The listing builds one solid part. Answer for the finished solid, in the listing's coordinates (mm). Coordinates: 2 decimals unless noted, no trailing zeros. Loops run counter-clockwise (first coordinate to the right, second up) from the corner with the lowest first, then second, coordinate; pieces in that order, holes last. Notation, with made-up numbers: (64.5, 51) - (96.5, 51) arc R17 ccw to (96.5, 78) - close; hole circle Ø3 at (66, 83). An arc over 180 degrees is marked (long way). Put each result on its own line as item: value.
```python
from build123d import *

# Parameters (mm, degrees)
F0_W          = 20
F0_H          = 75
F0_R          = 3.5
F1_DEPTH      = 1
F2_R          = 3
F3_DEPTH      = 75
F4_W          = 8
F4_H          = 15
F5_DEPTH      = 1.001
F5_DEPTH_BACK = 7.001


with BuildPart() as f1:
    # F0 (on Front) → F1 (new body)
    with BuildSketch(Plane.XZ):
        with Locations((-10, 0)):
            Rectangle(F0_W, F0_H)
        with Locations((-10, -26)):
            Circle(F0_R, mode=Mode.SUBTRACT)
        with Locations((-10, 0)):
            Circle(F0_R, mode=Mode.SUBTRACT)
        with Locations((-10, 26)):
            Circle(F0_R, mode=Mode.SUBTRACT)
    extrude(amount=F1_DEPTH)

    # F2 (on face) → F3 (join, through all)
    with BuildSketch(Plane(origin=(0, 0, -37.5), x_dir=(1, 0, 0), z_dir=(0, 0, -1))):
        with BuildLine():
            ThreePointArc((-20.8542486889, 1), (-19.8542486889, 2.3542486889), (-19.5, 4))
            ThreePointArc((-19.5, 4), (-26.3284271247, 6.8284271247), (-23.5, 0))
            ThreePointArc((-23.5, 0), (-22.0857864376, 0.2583426132), (-20.8542486889, 1))
        make_face()
        with Locations((-23.5, 4)):
            Circle(F2_R, mode=Mode.SUBTRACT)
        with BuildLine():
            ThreePointArc((-20.8542486889, 1), (-22.0857864376, 0.2583426132), (-23.5, 0))
            Line((-23.5, 0), (-20, 0))
            Line((-20, 0), (-20, 1))
            Line((-20, 1), (-20.8542486889, 1))
        make_face()
    extrude(amount=-F3_DEPTH)

    # F4 (on face) → F5 (cut, two sides)
    with BuildSketch(Plane.XZ.offset(1)) as f5_sk:
        with Locations((-23.5, 30)):
            Rectangle(F4_W, F4_H)
        with Locations((-23.5, -30)):
            Rectangle(F4_W, F4_H)
        with Locations((-23.5, 0)):
            Rectangle(F4_W, F4_H)
    extrude(amount=-F5_DEPTH, mode=Mode.SUBTRACT)
    extrude(f5_sk.sketch, amount=F5_DEPTH_BACK, mode=Mode.SUBTRACT)


solid = f1.part
```
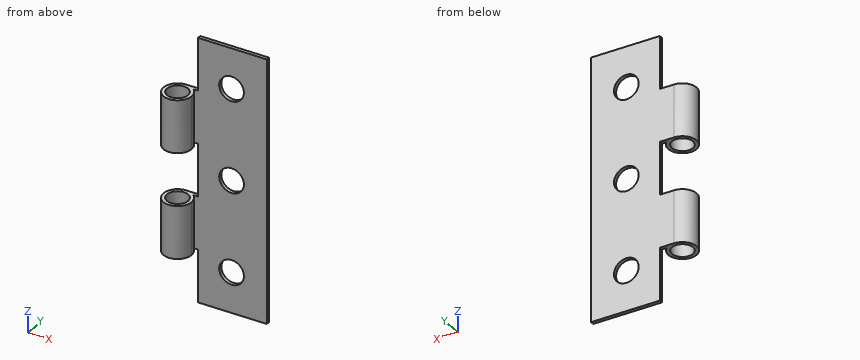
1) The part is cut by section D-D (z = 14). Give the vertices of the cut face in (x, y), and give its area (3 significant figures).
Found:
outline: (-23.5, 0) arc R4 ccw (long way) to (-20.85, -1) - (0, -1) - (0, 0) - close; hole circle Ø6 at (-23.5, -4)
area: 43.7 mm^2
2) Each of these flat-tipped pins is pushed along its axis until it touches: pin 1 (0.8 mm diameter, centred on y = -0.5, z = -31.5, fed in from -X); pin 2 (4 mm diameter, centred on x = -25, y = -4.5, fed in from -Z); pin 3 (4 mm diameter, centred on x = -10, z = 26, fed in from +Y); pin 4 (12 mm diameter, centred on x = -4, z = -13, fed in from -Y). Where does it stop, or does it pass through?
Found:
pin 1: stops at x = -19.5
pin 2: stops at z = -22.5
pin 3: passes through
pin 4: stops at y = -1
3) The part is cut by section C-C (y = -5.75). Give the vertices of the cut face in (x, z), and give its area (3 significant figures).
Found:
outline: (-27.1, -22.5) - (-25.94, -22.5) - (-25.94, -7.5) - (-27.1, -7.5) - close; (-27.1, 7.5) - (-25.94, 7.5) - (-25.94, 22.5) - (-27.1, 22.5) - close; (-21.06, -22.5) - (-19.9, -22.5) - (-19.9, -7.5) - (-21.06, -7.5) - close; (-21.06, 7.5) - (-19.9, 7.5) - (-19.9, 22.5) - (-21.06, 22.5) - close
area: 69.6 mm^2
4) Straight lines are drawn through the part: L1, parallel to Z at x = -10, y = -0.65; L2, parallel to Z at x = -24, y = -7; L3, parallel to Y at x = -23.5, z = 18. For each, find the intervals that lie inside material, in ascending order. Write a range as [from, to].
Found:
L1: z = [-37.5, -29.5], [-22.5, -3.5], [3.5, 22.5], [29.5, 37.5]
L2: z = [-22.5, -7.5], [7.5, 22.5]
L3: y = [-8, -7], [-1, 0]
5) The part is cut by section B-B (z = -26). Give the vertices of the cut face in (x, y).
Found:
outline: (-19.5, -1) - (-13.5, -1) - (-13.5, 0) - (-19.5, 0) - close; (-6.5, -1) - (0, -1) - (0, 0) - (-6.5, 0) - close
6) The part is cut by section A-A (x = -10). Give the vertices of the cut face in (y, z), and give its area (3 significant figures).
Found:
outline: (-1, -37.5) - (0, -37.5) - (0, -29.5) - (-1, -29.5) - close; (-1, -22.5) - (0, -22.5) - (0, -3.5) - (-1, -3.5) - close; (-1, 3.5) - (0, 3.5) - (0, 22.5) - (-1, 22.5) - close; (-1, 29.5) - (0, 29.5) - (0, 37.5) - (-1, 37.5) - close
area: 54.0 mm^2
